```python
from build123d import *

# Parameters (mm, degrees)
SKETCH1_W           = 42
SKETCH1_H           = 42
BOSS_EXTRUDE1_DEPTH = 9
CHAMFER1_SIZE       = 4
SKETCH2_R           = 4
CUT_EXTRUDE2_DEPTH  = 3
CUT_EXTRUDE2_TAPER  = -3


with BuildPart() as part:
    # Sketch1 → Boss-Extrude1 (new body)
    with BuildSketch(Plane(origin=(0, 0, 0), x_dir=(1, 0, 0), z_dir=(0, 1, 0))):
        Rectangle(SKETCH1_W, SKETCH1_H)
    extrude(amount=BOSS_EXTRUDE1_DEPTH)

    # Chamfer1
    chamfer1_edges = [part.edges().sort_by_distance(p)[0] for p in [
        (-21, 4.5, -21),
        (21, 4.5, -21),
        (21, 4.5, 21),
        (-21, 4.5, 21),
    ]]
    chamfer(chamfer1_edges, length=CHAMFER1_SIZE)

    # Sketch2 → Cut-Extrude2 (cut)
    with BuildSketch(Plane.XZ):
        Circle(SKETCH2_R)
    extrude(amount=-CUT_EXTRUDE2_DEPTH, taper=CUT_EXTRUDE2_TAPER, mode=Mode.SUBTRACT)


solid = part.part
```
Part model, mm, in its own coordinate system. A direction names the side the tool comes from. Round coordinates to 2 decimals unless told otherwise and drop trailing zeros. Loops run counter-clockwise (first coordinate to the right, second up) from the corner with the lowest first, then second, coordinate; pieces in that order, holes last.
1. Slice it at D-D (x = 18). Give the cut face in (y, z), and give its area (3 significant figures).
Solutions:
outline: (0, -20) - (9, -20) - (9, 20) - (0, 20) - close
area: 360 mm2
2. Two-plate mould, pull along X, no slides. Class faces 3 (the face through (0, 3, 0)), 4 (the face through (0, 4, -21)), 5 (the face through (-19, 4, -19)), 6 (the face through (19, 4, 19)): pulls with the +X half, pulls with the -X half, needs draft (parallel to the pull), parting line crosses it, or undercut.
Solutions:
face 3: undercut
face 4: needs draft
face 5: pulls with the -X half
face 6: pulls with the +X half
3. Slice it at A-A (y = 1). Give the cut face in (x, z), and give its area (3 significant figures).
Solutions:
outline: (-21, -17) - (-17, -21) - (17, -21) - (21, -17) - (21, 17) - (17, 21) - (-17, 21) - (-21, 17) - close; hole circle Ø8.1 at (0, 0)
area: 1,680 mm2
4. Slice it at C-C (y = 5.5). Give the cut face in (x, z).
Solutions:
outline: (-21, -17) - (-17, -21) - (17, -21) - (21, -17) - (21, 17) - (17, 21) - (-17, 21) - (-21, 17) - close
5. 3-axis set-ups, long thin cutter, end or side, ignore diameter. For faces 1 (the face through (3.875, 1.188, 1.22)), 2 (the face through (21, 4, 0)): which of +Z, -Z, +X, -X, +Y, -Y reach the whole face in a straight line?
Solutions:
face 1: none
face 2: +Z, -Z, +X, +Y, -Y
6. Slice it at B-B (x = 0). Give the cut face in (y, z), and give its area (3 significant figures).
Solutions:
outline: (0, -21) - (9, -21) - (9, 21) - (0, 21) - (0, 4) - (3, 4.16) - (3, -4.16) - (0, -4) - close
area: 354 mm2
7. Drill centre lines: line 1 along Z through (x, y) = (-17.5, 2.25); line 2 along X through (y, z) = (7.5, -18.5). Where is each one in solid material? Low to high.
Solutions:
line 1: z = -20.5 to 20.5
line 2: x = -19.5 to 19.5
8. Flat gauge pin, fed straight in: pin 1 (9 mm diameter, centred on x = 0, z = 0, fed in from -Y). Where does the tip first touch, or does it go through?
Solutions:
pin 1: stops at y = 0
